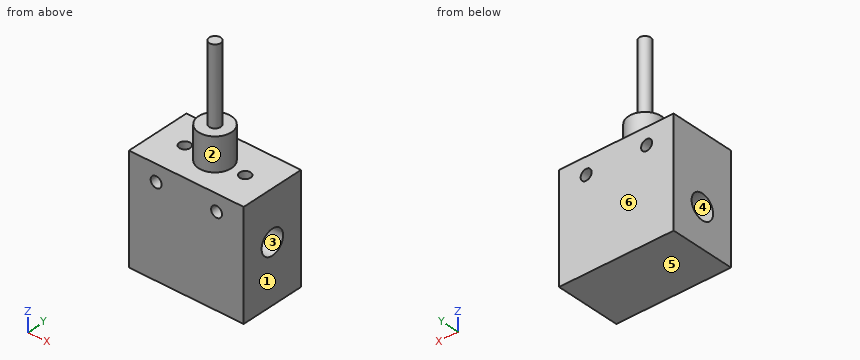
```python
from build123d import *

# Parameters (mm, degrees)
F0_W      = 66.548
F0_H      = 61.976
F1_DEPTH  = 19.05
F2_R      = 9.525
F2_R_2    = 3.302
F3_DEPTH  = 19.05
F3_FACE_R = 3.302
F4_DEPTH  = 63.5
F2_R_3    = 3.175
F5_DEPTH  = 9.652
F6_R      = 3.175
F7_DEPTH  = 38.101
F8_R      = 7.14375
F9_DEPTH  = 19.05
F10_R     = 7.14375
F11_DEPTH = 19.05


with BuildPart() as f1:
    # F0 (on Front) → F1 (new body, symmetric)
    with BuildSketch(Plane.XZ):
        Rectangle(F0_W, F0_H)
    extrude(amount=F1_DEPTH, both=True)

    # F2 (on face) → F3 (join)
    with BuildSketch(Plane.XY.offset(30.988)):
        Circle(F2_R)
        Circle(F2_R_2, mode=Mode.SUBTRACT)
    extrude(amount=F3_DEPTH)

    # F3_face (on face) → F4 (join)
    with BuildSketch(Plane.XY.offset(30.988)):
        Circle(F3_FACE_R)
    extrude(amount=F4_DEPTH)

    # F2 (on face) → F5 (cut)
    with BuildSketch(Plane.XY.offset(30.988)):
        with Locations((-17.526, 0)):
            Circle(F2_R_3)
        with Locations((17.526, 0)):
            Circle(F2_R_3)
    extrude(amount=-F5_DEPTH, mode=Mode.SUBTRACT)

    # F6 (on face) → F7 (cut, through all)
    with BuildSketch(Plane.XZ.offset(19.05)):
        with Locations((-17.526, 21.336)):
            Circle(F6_R)
        with Locations((17.526, 21.336)):
            Circle(F6_R)
    extrude(amount=-F7_DEPTH, mode=Mode.SUBTRACT)

    # F8 (on face) → F9 (cut)
    with BuildSketch(Plane.YZ.offset(33.274)):
        with Locations((0, 2.54)):
            Circle(F8_R)
    extrude(amount=-F9_DEPTH, mode=Mode.SUBTRACT)

    # F10 (on face) → F11 (cut)
    with BuildSketch(Plane(origin=(-33.274, 0, 0), x_dir=(0, -1, 0), z_dir=(-1, 0, 0))):
        with Locations((0, -8.636)):
            Circle(F10_R)
    extrude(amount=-F11_DEPTH, mode=Mode.SUBTRACT)


solid = f1.part
```
Verification items for the finished model (mm, model axes). Face numbers are marked on the shaded views. A direction names the side the tool comes from. Round coordinates to 2 decimals unless told otherwise and drop trailing zeros. Order: outer loops, then holes, each group sorted by start corner. A loop starts at its lowest first (then second) coordinate and runs counter-clockwise, first axis right, second up.
1) Draft check along Z on the marked faces 4, 5 and 6. Enter one of: +Z half, -Z half, draft (parallel to the pull), parting line (faces both ways), or undercut.
Geometry says:
face 4: undercut
face 5: -Z half
face 6: draft
2) Material ranges on line 1 (Z direction, x = 24, y = 0); line 2 (Z direction, x = -21, y = 0); line 3 (Z direction, x = 28, y = -16), recorded low to high.
Geometry says:
line 1: z = -30.99 to -4.6, 9.68 to 30.99
line 2: z = -30.99 to -15.78, -1.49 to 30.99
line 3: z = -30.99 to 30.99
3) Cross-section at D-D, the plane x = 28.5. Record the cut outline in (y, z).
Geometry says:
outline: (-19.05, -30.99) - (19.05, -30.99) - (19.05, 30.99) - (-19.05, 30.99) - close; hole circle Ø14.29 at (0, 2.54)
4) Cross-section at C-C, the plane y = 15.5. Record the cut outline in (x, z) (3 decimals).
Geometry says:
outline: (-33.274, -30.988) - (33.274, -30.988) - (33.274, 30.988) - (-33.274, 30.988) - close; hole circle Ø6.35 at (-17.526, 21.336); hole circle Ø6.35 at (17.526, 21.336)
5) Cross-section at B-B, the plane z = 2.54. Record the cut outline in (x, y), plus the area to 3 significant figures.
Geometry says:
outline: (-33.27, -19.05) - (33.27, -19.05) - (33.27, -7.14) - (14.22, -7.14) - (14.22, 7.14) - (33.27, 7.14) - (33.27, 19.05) - (-33.27, 19.05) - close
area: 2,260 mm2
6) Depth check by flat-ended pin: pin 1 (7 mm diameter, centred on y = -1, z = 0, fed in from +X); pin 2 (1.5 mm diameter, centred on x = -0.5, z = 34.5, fed in from +Y) (3 decimals); pin 3 (16.5 mm diameter, centred on y = 0, z = -8.636, fed in from -X); pin 4 (11.5 mm diameter, centred on y = 1, z = -8.5, fed in from -X). Enter the tip coordinate at first touch or a pass-through.
Geometry says:
pin 1: stops at x = 14.22
pin 2: stops at y = 9.525
pin 3: stops at x = -33.27
pin 4: stops at x = -14.22
7) Tool access check on the marked faces 1, 2 and 3. Record the directions out of +Z, -Z, +X, -X, +Y, -Y that give a thin tool (end or side, any length) a straight path to the whole face; none if there is none.
Geometry says:
face 1: +Z, -Z, +X, +Y, -Y
face 2: +Z
face 3: +X
8) Cross-section at A-A, the plane x = -16. Record the cut outline in (y, z), plus the area to 3 significant figures.
Geometry says:
outline: (-19.05, -30.99) - (19.05, -30.99) - (19.05, 18.55) - (-19.05, 18.55) - close; (-19.05, 24.12) - (-2.78, 24.12) - (-2.78, 30.99) - (-19.05, 30.99) - close; (2.78, 24.12) - (19.05, 24.12) - (19.05, 30.99) - (2.78, 30.99) - close; hole circle Ø14.29 at (0, -8.64)
area: 1,950 mm2
